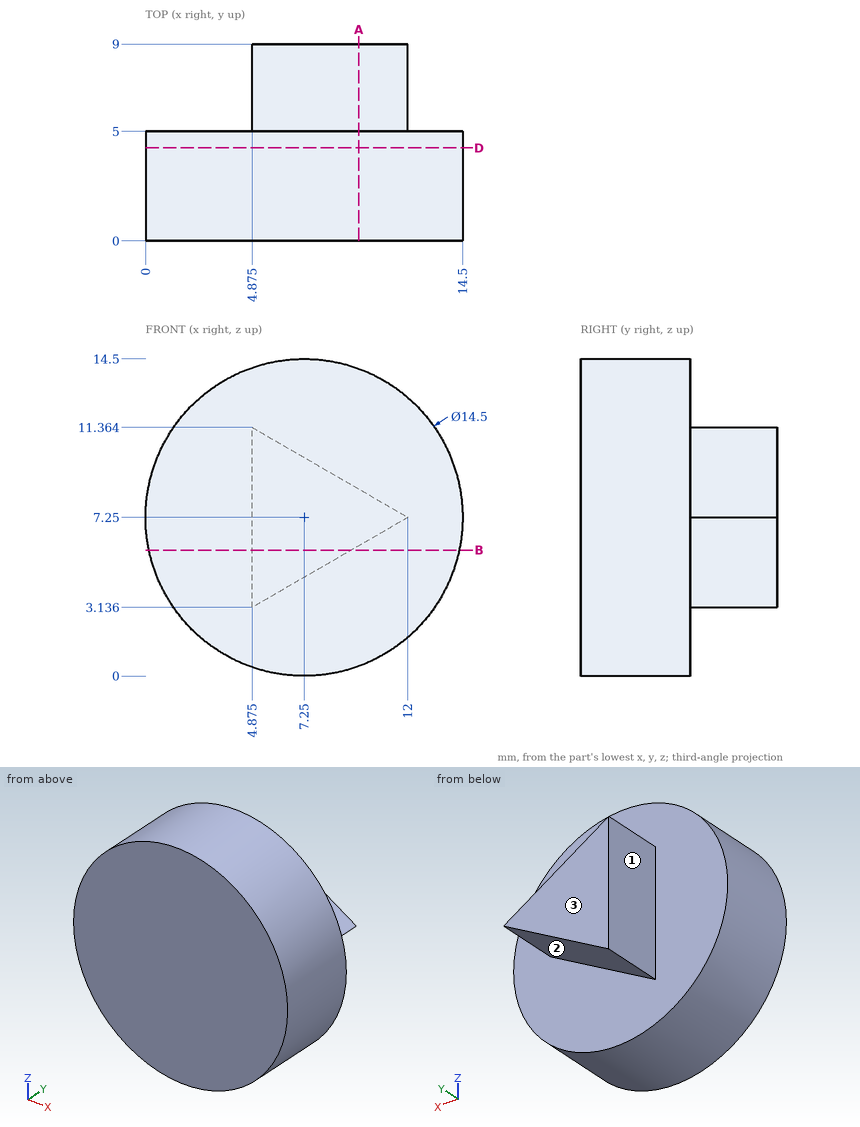
Verification items for this drawing (mm, ordinates from the low corner). A direction names the side the tool comes from. Coordinates: 2 decimals unless noted, no trailing zeros. Write each loop counter-clockwise with the first axis right and the second up, starting at its lowest first coordinate (ties: lowest second). Pieces come first, ordered by that corner, then holes. Notation, with made-up numbers: M 51,-38 L 63,-38 A24 cw 63,-12 Z; hole C -1.5,-7 d6. An arc over 180 degrees is marked long. Use one line per item in the form item = value. Start each with the question number.
1) Section check D-D on y = 4.25. Enter the section's corners in (x, z), and give its area (3 significant figures).
2) Section check A-A on x = 9.75. Enter the section's corners in (y, z) (1 decimal).
3) Go/stop test with flat-tipped pins: pin 1 Ø5 at (y, z) = (5, 2.5) entering from -X; pin 2 Ø4 at (y, z) = (6.5, 2.5) entering from +X; pin 3 Ø2 at (y, z) = (6.5, 5.5) entering from -X (3 decimals). Record where each tip stops, or that it passes through.
4) Set-up check for the marked faces 1, 2 and 3: record each of +Z, -Z, +X, -X, +Y, -Y from which the full face is reachable in a straight line by a thin tool's end or side.
5) Section check B-B on z = 5.75. Enter the section's corners in (x, y) (1 decimal).
6) Thickness scan on probe 1 along Y at (x, z) = (8.5, 12.75); probe 2 along X at (y, z) = (8.75, 5) (1 decimal); probe 3 along X at (y, z) = (4.5, 8.25). Record the ranges inside material, lowest first. Write a range as from..to.
Responses:
q1.outline = C 7.25,7.25 d14.5
q1.area = 165 mm2
q2.outline = M 0,0.4 L 5,0.4 L 5,6 L 9,6 L 9,8.5 L 5,8.5 L 5,14.1 L 0,14.1 Z
q3.pin_1 = 0.36
q3.pin_2 = 13.64
q3.pin_3 = 4.875
q4.face_1 = +Z, -Z, -X, +Y
q4.face_2 = -Z, +X, +Y
q4.face_3 = +Z, -Z, +X, -X, +Y
q5.outline = M 0.2,0 L 14.3,0 L 14.3,5 L 9.4,5 L 9.4,9 L 4.9,9 L 4.9,5 L 0.2,5 Z
q6.probe_1 = 0..5
q6.probe_2 = 4.9..8.1
q6.probe_3 = 0.07..14.43
